```python
from build123d import *

# Parameters (mm, degrees)
ESQUISSE2_W              = 105.34
ESQUISSE2_H              = 125.21
ESQUISSE2_W_2            = 101.44
ESQUISSE2_H_2            = 121.31
BASE_DEPTH               = 3
ESQUISSE3_R              = 4.5
SUPPORT_PCB_DEPTH        = 5
ESQUISSE4_R              = 2.25
ESQUISSE4_R_2            = 1.5
INSERT_M3_PCB_DEPTH      = 3
ESQUISSE4_3_R            = 1.5
PASSAGE_M3_PCB_DEPTH     = 5
ESQUISSE2_4_W            = 105.34
ESQUISSE2_4_H            = 125.21
ESQUISSE2_4_W_2          = 101.44
ESQUISSE2_4_H_2          = 121.31
WALLS_DEPTH              = 27
OUVERTURE_CONN_CMC_REACH = 140.494
ESQUISSE5_W              = 46.7
ESQUISSE5_H              = 20.1
CHANFREIN1_SIZE          = 12
CONG_1_R                 = 2
ESQUISSE6_R              = 2.25
INSERT_M3_BOX_DEPTH      = 3
ESQUISSE6_3_R            = 1.6
PASSAGE_M3_BOX_DEPTH     = 18
ESQUISSE10_R             = 3.1
BOSS_EXTRU_2_DEPTH       = 5
CONG_4_R                 = 5
PASSAGE_MAP_REACH        = 147.406
ESQUISSE11_R             = 3.5


with BuildPart() as part:
    # Esquisse2 → Base (new body)
    # profile 1 of 2: a face of its own
    with BuildSketch(Plane(origin=(0, 0, 0), x_dir=(1, 0, 0), z_dir=(0, 1, 0))):
        with Locations((0, -2.05)):
            Rectangle(ESQUISSE2_W, ESQUISSE2_H)
        with Locations((0, -2.05)):
            Rectangle(ESQUISSE2_W_2, ESQUISSE2_H_2, mode=Mode.SUBTRACT)
    # profile 2 of 2: a face of its own
    with BuildSketch(Plane(origin=(0, 0, 0), x_dir=(1, 0, 0), z_dir=(0, 1, 0))):
        with Locations((0, -2.05)):
            Rectangle(ESQUISSE2_W_2, ESQUISSE2_H_2)
    extrude(amount=-BASE_DEPTH)

    # Esquisse3 → Support_PCB (add)
    with BuildSketch(Plane(origin=(0, 0, 0), x_dir=(1, 0, 0), z_dir=(0, 1, 0))):
        with Locations(Location((-40.64, 47.117, 0), (0, 0, 270))):
            Circle(ESQUISSE3_R)
        with Locations(Location((40.64, 47.117, 0), (0, 0, 270))):
            Circle(ESQUISSE3_R)
        with Locations(Location((-40.64, -47.117, 0), (0, 0, 90))):
            Circle(ESQUISSE3_R)
        with Locations(Location((40.64, -47.117, 0), (0, 0, 90))):
            Circle(ESQUISSE3_R)
    extrude(amount=SUPPORT_PCB_DEPTH)

    # Esquisse4 → Insert_M3_PCB (cut)
    # profile 1 of 8: a face of its own
    with BuildSketch(Plane(origin=(0, 5, 0), x_dir=(1, 0, 0), z_dir=(0, 1, 0))):
        with Locations(Location((-40.64, 47.117, 0), (0, 0, 270))):
            Circle(ESQUISSE4_R)
        with Locations((-40.64, 47.117)):
            Circle(ESQUISSE4_R_2, mode=Mode.SUBTRACT)
    # profile 2 of 8: a face of its own
    with BuildSketch(Plane(origin=(0, 5, 0), x_dir=(1, 0, 0), z_dir=(0, 1, 0))):
        with Locations((-40.64, 47.117)):
            Circle(ESQUISSE4_R_2)
    # profile 3 of 8: a face of its own
    with BuildSketch(Plane(origin=(0, 5, 0), x_dir=(1, 0, 0), z_dir=(0, 1, 0))):
        with Locations(Location((40.64, 47.117, 0), (0, 0, 270))):
            Circle(ESQUISSE4_R)
        with Locations((40.64, 47.117)):
            Circle(ESQUISSE4_R_2, mode=Mode.SUBTRACT)
    # profile 4 of 8: a face of its own
    with BuildSketch(Plane(origin=(0, 5, 0), x_dir=(1, 0, 0), z_dir=(0, 1, 0))):
        with Locations((40.64, 47.117)):
            Circle(ESQUISSE4_R_2)
    # profile 5 of 8: a face of its own
    with BuildSketch(Plane(origin=(0, 5, 0), x_dir=(1, 0, 0), z_dir=(0, 1, 0))):
        with Locations(Location((40.64, -47.117, 0), (0, 0, 270))):
            Circle(ESQUISSE4_R)
        with Locations((40.64, -47.117)):
            Circle(ESQUISSE4_R_2, mode=Mode.SUBTRACT)
    # profile 6 of 8: a face of its own
    with BuildSketch(Plane(origin=(0, 5, 0), x_dir=(1, 0, 0), z_dir=(0, 1, 0))):
        with Locations((40.64, -47.117)):
            Circle(ESQUISSE4_R_2)
    # profile 7 of 8: a face of its own
    with BuildSketch(Plane(origin=(0, 5, 0), x_dir=(1, 0, 0), z_dir=(0, 1, 0))):
        with Locations(Location((-40.64, -47.117, 0), (0, 0, 270))):
            Circle(ESQUISSE4_R)
        with Locations((-40.64, -47.117)):
            Circle(ESQUISSE4_R_2, mode=Mode.SUBTRACT)
    # profile 8 of 8: a face of its own
    with BuildSketch(Plane(origin=(0, 5, 0), x_dir=(1, 0, 0), z_dir=(0, 1, 0))):
        with Locations((-40.64, -47.117)):
            Circle(ESQUISSE4_R_2)
    extrude(amount=-INSERT_M3_PCB_DEPTH, mode=Mode.SUBTRACT)

    # Esquisse4<3> → Passage M3_PCB (cut)
    with BuildSketch(Plane(origin=(0, 5, 0), x_dir=(1, 0, 0), z_dir=(0, 1, 0))):
        with Locations(Location((-40.64, -47.117, 0), (0, 0, 270))):
            Circle(ESQUISSE4_3_R)
        with Locations(Location((40.64, -47.117, 0), (0, 0, 270))):
            Circle(ESQUISSE4_3_R)
        with Locations(Location((40.64, 47.117, 0), (0, 0, 270))):
            Circle(ESQUISSE4_3_R)
        with Locations(Location((-40.64, 47.117, 0), (0, 0, 270))):
            Circle(ESQUISSE4_3_R)
    extrude(amount=-PASSAGE_M3_PCB_DEPTH, mode=Mode.SUBTRACT)

    # Esquisse2<4> → Walls (add)
    with BuildSketch(Plane(origin=(0, 0, 0), x_dir=(1, 0, 0), z_dir=(0, 1, 0))):
        with Locations((0, -2.05)):
            Rectangle(ESQUISSE2_4_W, ESQUISSE2_4_H)
        with Locations((0, -2.05)):
            Rectangle(ESQUISSE2_4_W_2, ESQUISSE2_4_H_2, mode=Mode.SUBTRACT)
    extrude(amount=WALLS_DEPTH)

    # Esquisse5 → Ouverture_Conn_CMC (cut, up to next)
    with BuildSketch(Plane(origin=(0, 0, -60.555), x_dir=(-1, 0, 0), z_dir=(0, 0, -1)), mode=Mode.PRIVATE) as ouverture_conn_cmc_sk1:
        with Locations((0, 16.95)):
            Rectangle(ESQUISSE5_W, ESQUISSE5_H)
    ouverture_conn_cmc_tool1 = extrude(ouverture_conn_cmc_sk1.sketch, amount=-OUVERTURE_CONN_CMC_REACH, mode=Mode.PRIVATE) & part.part
    add(ouverture_conn_cmc_tool1.solids().sort_by_distance((0, 16.95, -60.555))[0], mode=Mode.SUBTRACT)

    # Chanfrein1
    chanfrein1_edges = [part.edges().sort_by_distance(p)[0] for p in [
        (-50.72, 13.5, -58.605),
        (50.72, 13.5, -58.605),
        (50.72, 13.5, 62.705),
        (-50.72, 13.5, 62.705),
    ]]
    chamfer(chanfrein1_edges, length=CHANFREIN1_SIZE)

    # Congé1
    cong_1_edges = [part.edges().sort_by_distance(p)[0] for p in [
        (0, 0, -58.605),
        (50.72, 0, 2.05),
        (-50.72, 0, 2.05),
        (0, 0, 62.705),
        (-40.64, 0, -51.617),
        (40.64, 0, -51.617),
        (-40.64, 0, 51.617),
        (40.64, 0, 51.617),
        (52.67, 12, -60.555),
        (52.67, 12, 64.655),
        (-52.67, 12, 64.655),
        (-52.67, 12, -60.555),
    ]]
    fillet(cong_1_edges, radius=CONG_1_R)

    # Esquisse6 → Insert_M3_Box (cut)
    with BuildSketch(Plane(origin=(0, 27, 0), x_dir=(1, 0, 0), z_dir=(0, 1, 0))):
        with Locations(Location((-47.598784258, 55.483784258, 0), (0, 0, 270))):
            Circle(ESQUISSE6_R)
        with Locations(Location((-47.598784258, -59.583784258, 0), (0, 0, 270))):
            Circle(ESQUISSE6_R)
        with Locations(Location((47.598784258, 55.483784258, 0), (0, 0, 270))):
            Circle(ESQUISSE6_R)
        with Locations(Location((47.598784258, -59.583784258, 0), (0, 0, 270))):
            Circle(ESQUISSE6_R)
    extrude(amount=-INSERT_M3_BOX_DEPTH, mode=Mode.SUBTRACT)

    # Esquisse6<3> → Passage_M3_Box (cut)
    with BuildSketch(Plane(origin=(0, 27, 0), x_dir=(1, 0, 0), z_dir=(0, 1, 0))):
        with Locations(Location((-47.598784258, 55.483784258, 0), (0, 0, 270))):
            Circle(ESQUISSE6_3_R)
        with Locations(Location((-47.598784258, -59.583784258, 0), (0, 0, 270))):
            Circle(ESQUISSE6_3_R)
        with Locations(Location((47.598784258, 55.483784258, 0), (0, 0, 270))):
            Circle(ESQUISSE6_3_R)
        with Locations(Location((47.598784258, -59.583784258, 0), (0, 0, 270))):
            Circle(ESQUISSE6_3_R)
    extrude(amount=-PASSAGE_M3_BOX_DEPTH, mode=Mode.SUBTRACT)

    # Esquisse10 → Boss.-Extru.2 (add)
    # profile 1 of 2: a face of its own
    with BuildSketch(Plane.XZ.offset(3)):
        with BuildLine():
            Line((52.67, 25), (72.67, 5))
            ThreePointArc((72.67, 5), (74.741067812, 0), (72.67, -5))
            Line((72.67, -5), (52.67, -25))
            Line((52.67, -25), (52.67, 25))
        make_face()
        with Locations(Location((64.67, 0, 0), (0, 0, 270))):
            Circle(ESQUISSE10_R, mode=Mode.SUBTRACT)
    # profile 2 of 2: a face of its own
    with BuildSketch(Plane.XZ.offset(3)):
        with BuildLine():
            Line((-52.67, 25), (-72.67, 5))
            ThreePointArc((-72.67, 5), (-74.741067812, 0), (-72.67, -5))
            Line((-72.67, -5), (-52.67, -25))
            Line((-52.67, -25), (-52.67, 25))
        make_face()
        with Locations(Location((-64.67, 0, 0), (0, 0, 90))):
            Circle(ESQUISSE10_R, mode=Mode.SUBTRACT)
    extrude(amount=-BOSS_EXTRU_2_DEPTH)

    # Congé4
    cong_4_edges = [part.edges().sort_by_distance(p)[0] for p in [
        (52.67, 2, 0),
        (52.67, -0.5, -25),
        (52.67, -0.5, 25),
        (-52.67, 2, 0),
        (-52.67, -0.5, 25),
        (-52.67, -0.5, -25),
    ]]
    fillet(cong_4_edges, radius=CONG_4_R)

    # Esquisse11 → Passage_MAP (cut, up to next)
    with BuildSketch(Plane(origin=(52.67, 0, 0), x_dir=(0, 0, -1), z_dir=(1, 0, 0)), mode=Mode.PRIVATE) as passage_map_sk1:
        with Locations((-36.375, 12.6)):
            Circle(ESQUISSE11_R)
    passage_map_tool1 = extrude(passage_map_sk1.sketch, amount=-PASSAGE_MAP_REACH, mode=Mode.PRIVATE) & part.part
    add(passage_map_tool1.solids().sort_by_distance((52.67, 12.6, 36.375))[0], mode=Mode.SUBTRACT)


solid = part.part
```
Build history of the part. All positions in model axes, mm. A direction names the side the tool comes from. Coordinates: 2 decimals unless noted, no trailing zeros. Order: outer loops, then holes, each group sorted by start corner. A loop starts at its lowest first (then second) coordinate and runs counter-clockwise, first axis right, second up. Notation, with made-up numbers: M -17.75,79.25 L -10.75,79.25 A16 cw -10.75,95.25 Z; hole C 60,3.5 d9. An arc over 180 degrees is marked long. One line per question, with ' | ' between items. Start each with the question number.
1. Flat gauge pins, fed straight in: P1, Ø2.5, axis at x = -43, z = 45.5, coming from the +Y side; P2, Ø1.6, axis at x = -48, z = -55, coming from the +Y side; P3, Ø15, axis at y = 10, z = -23, coming from the +X side. Where does each tip first touch, or does it go through?
2. Cut at C-C (y = 12.6). Write the cut outline in (x, z) (3 decimals), plus the area to 3 significant figures.
3. Mould opens along Z. For faces 3 (the face through (39.288, 3.479, 42.825)), 4 (the face through (52.67, 15, 3)), 5 (the face through (-63.53, -0.53, -14.14)), 6 (the face through (-41, 2, -49)) say: +Z half, -Z half, draft (parallel to the pull), parting line (faces both ways), or undercut.
4. Cut at B-B (z = 0). Write the cut outline in (x, y).
5. Tool access for faces 1 (the face through (46.6, 24, 61.1)), 2 (the face through (53.04, 0.96, -25.18)): list every direction of +Z, -Z, +X, -X, +Y, -Y with a clear straight run to the whole face (end or side of a thin tool).
6. Cut at A-A (x = -64.67). Write the cut outline in (y, z).
7. Wall check: line 1 along X through (y, z) = (17.5, 35); line 2 along X through (y, z) = (2.5, -46); line 3 along X through (y, z) = (13.5, -55) (3 decimals). Give the ranges that are in metal, low to high. Write a range as [from, to].
The answers:
1) P1: stops at y = 5 | P2: stops at y = 9 | P3: stops at x = 55.42
2) outline: M -52.67,-58.555 A2 ccw -50.67,-60.555 L -23.35,-60.555 L -23.35,-58.605 L -38.72,-58.605 L -50.72,-46.605 L -50.72,50.705 L -38.72,62.705 L 38.72,62.705 L 50.72,50.705 L 50.72,39.875 L 52.67,39.875 L 52.67,62.655 A2 ccw 50.67,64.655 L -50.67,64.655 A2 ccw -52.67,62.655 Z; M 23.35,-60.555 L 50.67,-60.555 A2 ccw 52.67,-58.555 L 52.67,32.875 L 50.72,32.875 L 50.72,-46.605 L 38.72,-58.605 L 23.35,-58.605 Z; hole C -47.599,-55.484 d3.2; hole C -47.599,59.584 d3.2; hole C 47.599,-55.484 d3.2; hole C 47.599,59.584 d3.2 | area: 1,030 mm2
3) face 3: undercut | face 4: draft | face 5: -Z half | face 6: undercut
4) outline: M -74.74,-3 L -67.77,-3 L -67.77,2 L -74.74,2 Z; M -61.57,-3 L 61.57,-3 L 61.57,2 L 57.67,2 A5 cw 52.67,7 L 52.67,27 L 50.72,27 L 50.72,2 A2 cw 48.72,0 L -48.72,0 A2 cw -50.72,2 L -50.72,27 L -52.67,27 L -52.67,7 A5 cw -57.67,2 L -61.57,2 Z; M 67.77,-3 L 74.74,-3 L 74.74,2 L 67.77,2 Z
5) face 1: +Y | face 2: -Z, +X, +Y, -Y
6) outline: M -3,-13 L 2,-13 L 2,-3.1 L -3,-3.1 Z; M -3,3.1 L 2,3.1 L 2,13 L -3,13 Z
7) line 1: x = [-52.67, -50.72], [50.72, 52.67] | line 2: x = [-52.67, -50.72], [-45, -42.59], [-38.69, -36.28], [36.28, 38.69], [42.59, 45], [50.72, 52.67] | line 3: x = [-52.67, -49.124], [-46.074, -42.325], [42.325, 46.074], [49.124, 52.67]
